Geometry check sheet. Reference: drawing and pictorial views, mm from the part's lowest x, y, z. A direction names the side the tool comes from. Give positions to 0.01 mm unless a question says otherwise; leave off trailing zeros. Order: outer loops, then holes, each group sorted by start corner. A loop starts at its lowest first (then second) coordinate and runs counter-clockwise, first axis right, second up. Notation, with made-up numbers: (23, 8.25) - (75, 8.25) arc R9 cw to (75, 24.25) - close; hole circle Ø4 at (7, 33). An arc over 180 degrees is marked (long way). Answer in a Markdown table with one row per item.
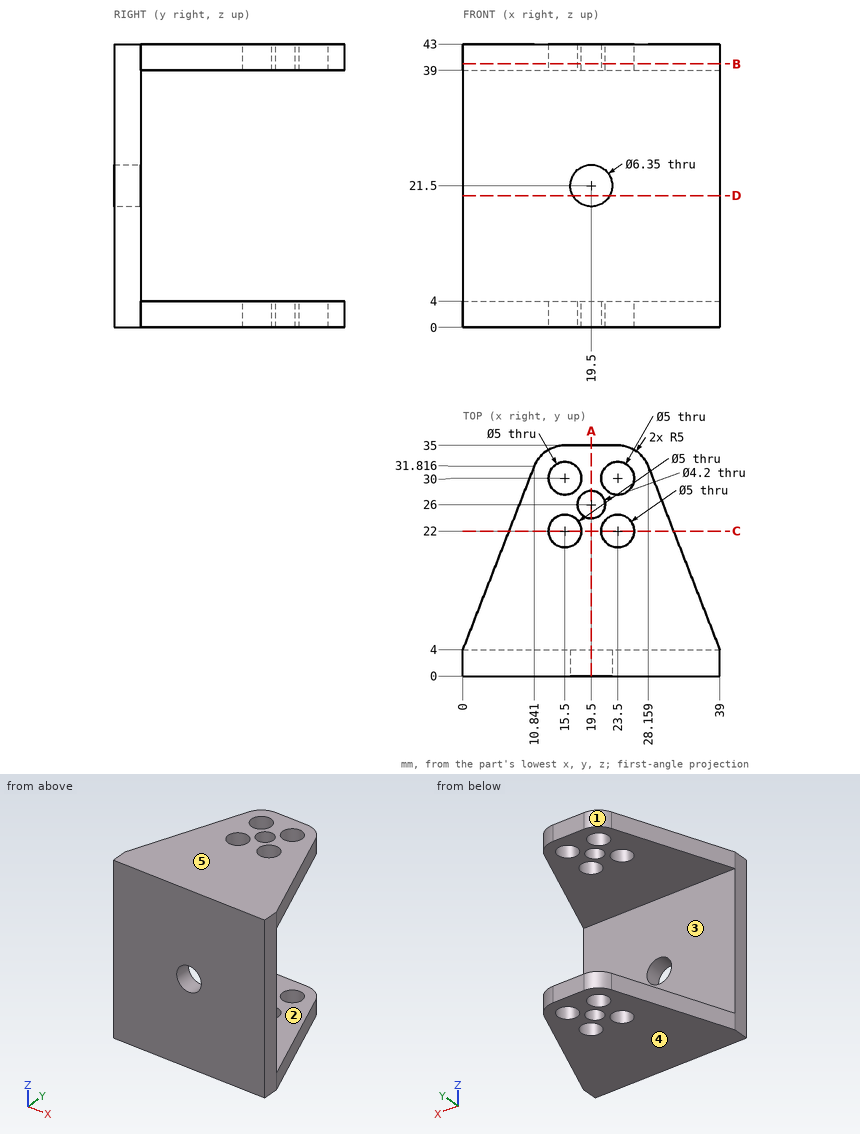
(1) Gauge pin test, flat ends, axial feed: P1, Ø8, axis at x = 23.5, y = 22, coming from the +Z side; P2, Ø6, axis at y = 26.5, z = 4.5, coming from the -X side; P3, Ø8, axis at x = 28, z = 20.5, coming from the +Y side. Record the tip position at first contact, or that the pin passes through.
Geometry says:
| item | result |
|---|---|
| P1 | z = 43 |
| P2 | x = 7.62 |
| P3 | y = 4 |
(2) Cross-section at C-C, the plane y = 22. Record the cut outline in (x, z) (1 decimal), then the cut area to 3 significant figures.
Geometry says:
| item | result |
|---|---|
| outline | (7, 0) - (13, 0) - (13, 4) - (7, 4) - close; (7, 39) - (13, 39) - (13, 43) - (7, 43) - close; (18, 0) - (21, 0) - (21, 4) - (18, 4) - close; (18, 39) - (21, 39) - (21, 43) - (18, 43) - close; (26, 0) - (32, 0) - (32, 4) - (26, 4) - close; (26, 39) - (32, 39) - (32, 43) - (26, 43) - close |
| area | 120 mm² |
(3) Cross-section at A-A, the plane x = 19.5. Record the cut outline in (y, z) (1 decimal), then the cut area to 3 significant figures.
Geometry says:
| item | result |
|---|---|
| outline | (0, 0) - (23.9, 0) - (23.9, 4) - (4, 4) - (4, 18.3) - (0, 18.3) - close; (0, 24.7) - (4, 24.7) - (4, 39) - (23.9, 39) - (23.9, 43) - (0, 43) - close; (28.1, 0) - (35, 0) - (35, 4) - (28.1, 4) - close; (28.1, 39) - (35, 39) - (35, 43) - (28.1, 43) - close |
| area | 361 mm² |
(4) Mould release check, pull along Z, two halves, no side actions. Record for the marked faces 3, 4 and 5: pulls with the +Z half, pulls with the -Z half, needs draft (parallel to the pull), parting line crosses it, or undercut.
Geometry says:
| item | result |
|---|---|
| face 3 | undercut |
| face 4 | pulls with the -Z half |
| face 5 | pulls with the +Z half |
(5) Thickness scan on L1, parallel to Z at x = 18, y = 31; L2, parallel to Y at x = 19.5, z = 41.1; L3, parallel to X at y = 30, z = 1. Record the ranges inside material, lowest first.
Geometry says:
| item | result |
|---|---|
| L1 | 0 to 4, 39 to 43 |
| L2 | 0 to 23.9, 28.1 to 35 |
| L3 | 10.13 to 13, 18 to 21, 26 to 28.87 |
(6) Cross-section at B-B, the plane z = 40. Record the cut outline in (x, y), then the cut area to 3 significant figures.
Geometry says:
| item | result |
|---|---|
| outline | (0, 0) - (39, 0) - (39, 4) - (28.16, 31.82) arc R5 ccw to (23.5, 35) - (15.5, 35) arc R5 ccw to (10.84, 31.82) - (0, 4) - close; hole circle Ø5 at (15.5, 22); hole circle Ø5 at (15.5, 30); hole circle Ø4.2 at (19.5, 26); hole circle Ø5 at (23.5, 22); hole circle Ø5 at (23.5, 30) |
| area | 894 mm² |
(7) Cross-section at D-D, the plane z = 20. Record the cut outline in (x, y), then the cut area to 3 significant figures.
Geometry says:
| item | result |
|---|---|
| outline | (0, 0) - (16.7, 0) - (16.7, 4) - (0, 4) - close; (22.3, 0) - (39, 0) - (39, 4) - (22.3, 4) - close |
| area | 134 mm² |
(8) Access from +Z, -Z, +X, -X, +Y, -Y to the whole of each face (thin tool, end or side, straight path). Record for the marked faces 1 and 2.
Geometry says:
| item | result |
|---|---|
| face 1 | +Z, -Z, -X, +Y |
| face 2 | +X, -X, +Y |
